from build123d import *

# Parameters (mm, degrees)
SKETCH1_R           = 22.225
BOSS_EXTRUDE1_DEPTH = 91.44
CUT_EXTRUDE1_REACH  = 106.072
SKETCH2_W           = 4.445
SKETCH2_H           = 40.64
SKETCH4_R           = 1.905
CUT_EXTRUDE2_DEPTH  = 103.252746907
SKETCH6_W           = 44.45
SKETCH6_H           = 19.05
CUT_EXTRUDE3_DEPTH  = 685.739656498


with BuildPart() as part:
    # Sketch1 → Boss-Extrude1 (new body)
    with BuildSketch(Plane(origin=(0, 0, 0), x_dir=(1, 0, 0), z_dir=(0, 1, 0))):
        with Locations(Location((0, 0, 0), (0, 0, 270))):
            Circle(SKETCH1_R)
    extrude(amount=BOSS_EXTRUDE1_DEPTH)

    # Sketch2 → Cut-Extrude1 (cut, up to next)
    with BuildSketch(Plane(origin=(22.225, 0, 0), x_dir=(0, 0, -1), z_dir=(1, 0, 0)), mode=Mode.PRIVATE) as cut_extrude1_sk1:
        with Locations((-20.0025, 71.12)):
            Rectangle(SKETCH2_W, SKETCH2_H)
    cut_extrude1_tool1 = extrude(cut_extrude1_sk1.sketch, amount=-CUT_EXTRUDE1_REACH, mode=Mode.PRIVATE) & part.part
    # Sketch2 → Cut-Extrude1 (cut, up to next)
    with BuildSketch(Plane(origin=(22.225, 0, 0), x_dir=(0, 0, -1), z_dir=(1, 0, 0)), mode=Mode.PRIVATE) as cut_extrude1_sk2:
        with Locations((20.0025, 71.12)):
            Rectangle(SKETCH2_W, SKETCH2_H)
    cut_extrude1_tool2 = extrude(cut_extrude1_sk2.sketch, amount=-CUT_EXTRUDE1_REACH, mode=Mode.PRIVATE) & part.part
    add(cut_extrude1_tool1.solids().sort_by_distance((22.225, 71.12, 20.0025))[0], mode=Mode.SUBTRACT)
    add(cut_extrude1_tool2.solids().sort_by_distance((22.225, 71.12, -20.0025))[0], mode=Mode.SUBTRACT)

    # Sketch4 → Cut-Extrude2 (cut, through all)
    with BuildSketch(Plane.XY.offset(17.78)):
        with Locations((0, 74.93)):
            Circle(SKETCH4_R)
        with Locations((0, 63.5)):
            Circle(SKETCH4_R)
    extrude(amount=-CUT_EXTRUDE2_DEPTH, mode=Mode.SUBTRACT)

    # Sketch6 → Cut-Extrude3 (cut, through all)
    with BuildSketch(Plane(origin=(-69.793368373, -6.35, 649.219810065), x_dir=(0, 0, -1), z_dir=(1, 0, 0))):
        with Locations((649.219810065, 15.875)):
            Rectangle(SKETCH6_W, SKETCH6_H)
    extrude(amount=CUT_EXTRUDE3_DEPTH, mode=Mode.SUBTRACT)


solid = part.part
Build history of the part. All positions in model axes, mm. A direction names the side the tool comes from. Coordinates: 2 decimals unless noted, no trailing zeros. Order: outer loops, then holes, each group sorted by start corner. A loop starts at its lowest first (then second) coordinate and runs counter-clockwise, first axis right, second up. Notation, with made-up numbers: (-32.75, 71.5) - (5.25, 71.5) arc R22 cw to (5.25, 87.5) - close; hole circle Ø3 at (25, -38.75). An arc over 180 degrees is marked (long way). Write each question's results on one line, items separated by ' | '. Start each with the question number.
Item 1: Band-saw the part on B-B on y = 74.93. Write the cut outline in (x, z) (3 decimals).
Item 2: Band-saw the part on A-A on x = 0. Write the cut outline in (y, z) (3 decimals).
Item 3: Mould opens along X. For faces 1 (the face through (0, 19.05, 0)), 2 (the face through (0.977, 46.695, -22.204)), 3 (the face through (-0.41, 73.07, 0.25)) say: released by +X, released by -X, zero draft, split by the parting line, or undercut.
Item 4: Tool access for faces 4 (the face through (0, 91.44, 0)), 5 (the face through (0, 50.8, -19)), 6 (the face through (0, 50.8, 20)): list every direction of +Z, -Z, +X, -X, +Y, -Y with a clear straight run to the whole face (end or side of a thin tool).
Item 5: Flat gauge pins, fed straight in: pin 1 (1 mm diameter, centred on y = 68.5, z = 15, fed in from +X); pin 2 (21.5 mm diameter, centred on x = 5.5, y = 75.5, fed in from -Z); pin 3 (4.5 mm diameter, centred on x = 0, y = 74.93, fed in from +Z). Where does each tip first touch, or does it go through?
Item 6: Band-saw the part on D-D on y = 60. Write the cut outline in (x, z) (3 decimals), and give its area (3 significant figures).
Item 7: Band-saw the part on C-C on z = 9. Write the cut outline in (x, y) (3 decimals), and give its area (3 significant figures).
Item 8: Wall check: probe 1 along Y at (x, z) = (0, -7) (3 decimals); probe 2 along Z at (x, y) = (11.5, 74); probe 3 along X at (y, z) = (74.93, 7.5) (3 decimals). Give the ranges that are in metal, low to high. Write a range as [from, to].
Numbers:
1) outline: (-13.335, -17.78) - (-1.905, -17.78) - (-1.905, 17.78) - (-13.335, 17.78) arc R22.225 ccw to start; (1.905, -17.78) - (13.335, -17.78) arc R22.225 ccw to (13.335, 17.78) - (1.905, 17.78) - close
2) outline: (19.05, -22.225) - (50.8, -22.225) - (50.8, -17.78) - (61.595, -17.78) - (61.595, 17.78) - (50.8, 17.78) - (50.8, 22.225) - (19.05, 22.225) - close; (65.405, -17.78) - (73.025, -17.78) - (73.025, 17.78) - (65.405, 17.78) - close; (76.835, -17.78) - (91.44, -17.78) - (91.44, 17.78) - (76.835, 17.78) - close
3) face 1: zero draft | face 2: split by the parting line | face 3: undercut
4) face 4: +Z, -Z, +X, -X, +Y | face 5: -Z, +X, -X, +Y | face 6: +Z, +X, -X, +Y
5) pin 1: x = 16.84 | pin 2: z = -17.78 | pin 3: z = 17.78
6) outline: (-13.335, -17.78) - (13.335, -17.78) arc R22.225 ccw to (13.335, 17.78) - (-13.335, 17.78) arc R22.225 ccw to start | area: 1,390 mm^2
7) outline: (-20.321, 19.05) - (20.321, 19.05) - (20.321, 91.44) - (-20.321, 91.44) - close; hole circle Ø3.81 at (0, 63.5); hole circle Ø3.81 at (0, 74.93) | area: 2,920 mm^2
8) probe 1: [19.05, 61.595], [65.405, 73.025], [76.835, 91.44] | probe 2: [-17.78, 17.78] | probe 3: [-20.921, -1.905], [1.905, 20.921]
